```python
from build123d import *

# Parameters (mm, degrees)
BOSS_EXTRUDE2_DEPTH = 57.5
FILLET1_R           = 0.4
FILLET2_R           = 0.5
SKETCH5_R           = 4.25
CUT_EXTRUDE1_DEPTH  = 3
SKETCH6_R           = 3.25
CUT_EXTRUDE2_DEPTH  = 5.9
SKETCH7_R           = 4.25
CUT_EXTRUDE3_DEPTH  = 8
SKETCH8_R           = 3.25
CUT_EXTRUDE4_DEPTH  = 0.9
SKETCH9_W           = 30
SKETCH9_H           = 4.9
BOSS_EXTRUDE3_DEPTH = 2
CHAMFER1_SIZE       = 0.5


with BuildPart() as part:
    # Sketch4 → Boss-Extrude2 (new, symmetric)
    with BuildSketch(Plane(origin=(0, 0, 0), x_dir=(0, 0, -1), z_dir=(1, 0, 0))):
        Polygon((-15, 5), (15, 5), (15, 0.1), (5.883419246, 0.1), (8.770170592, -4.9), (-8.770170592, -4.9), (-5.883419246, 0.1), (-15, 0.1), align=None)
    extrude(amount=BOSS_EXTRUDE2_DEPTH, both=True)

    # Fillet1
    fillet1_edges = [part.edges().sort_by_distance(p)[0] for p in [
        (0, -4.9, -8.770170592),
        (0, -4.9, 8.770170592),
    ]]
    fillet(fillet1_edges, radius=FILLET1_R)

    # Fillet2
    fillet2_edges = [part.edges().sort_by_distance(p)[0] for p in [
        (0, 0.1, -5.883419246),
        (0, 0.1, 5.883419246),
    ]]
    fillet(fillet2_edges, radius=FILLET2_R)

    # Sketch5 → Cut-Extrude1 (cut)
    with BuildSketch(Plane.XZ.offset(4.9)):
        with Locations(Location((51.5, 0, 0), (0, 0, 270))):
            Circle(SKETCH5_R)
    extrude(amount=-CUT_EXTRUDE1_DEPTH, mode=Mode.SUBTRACT)

    # Sketch6 → Cut-Extrude2 (cut)
    with BuildSketch(Plane(origin=(0, 5, 0), x_dir=(1, 0, 0), z_dir=(0, 1, 0))):
        with Locations(Location((51.5, 0, 0), (0, 0, 270))):
            Circle(SKETCH6_R)
    extrude(amount=-CUT_EXTRUDE2_DEPTH, mode=Mode.SUBTRACT)

    # Sketch7 → Cut-Extrude3 (cut)
    with BuildSketch(Plane.XZ.offset(4.9)):
        with Locations(Location((-51.5, 0, 0), (0, 0, 270))):
            Circle(SKETCH7_R)
    extrude(amount=-CUT_EXTRUDE3_DEPTH, mode=Mode.SUBTRACT)

    # Sketch8 → Cut-Extrude4 (cut)
    with BuildSketch(Plane(origin=(0, 5, 0), x_dir=(1, 0, 0), z_dir=(0, 1, 0))):
        with Locations(Location((-51.5, 0, 0), (0, 0, 270))):
            Circle(SKETCH8_R)
    extrude(amount=-CUT_EXTRUDE4_DEPTH, mode=Mode.SUBTRACT)

    # Sketch9 → Boss-Extrude3 (add)
    with BuildSketch(Plane(origin=(57.5, 0, 0), x_dir=(0, 0, -1), z_dir=(1, 0, 0))):
        with Locations((0, 2.55)):
            Rectangle(SKETCH9_W, SKETCH9_H)
    extrude(amount=BOSS_EXTRUDE3_DEPTH)

    # Chamfer1
    chamfer1_edges = [part.edges().sort_by_distance(p)[0] for p in [
        (51.5, -4.9, 4.25),
        (-51.5, -4.9, 4.25),
    ]]
    chamfer(chamfer1_edges, length=CHAMFER1_SIZE)


solid = part.part
```
Could you check a few things on this model? Use its own coordinates, in mm. A direction names the side the tool comes from. Coordinates: 2 decimals unless noted, no trailing zeros. Write each loop counter-clockwise with the first axis right and the second up, starting at its lowest first coordinate (ties: lowest second). Pieces come first, ordered by that corner, then holes. Notation, with made-up numbers: (46.25, 7.5) - (82.25, 7.5) arc R21 ccw to (82.25, 31.5) - close; hole circle Ø11 at (5, 51). An arc over 180 degrees is marked (long way). Use a Markdown table: item, result.
Q1. Imagine slicing it at C-C (x = -51.5). List the corners of the cut face in (y, z) for me.
Geometry check:
| item | result |
|---|---|
| outline | (-4.9, -8.08) arc R0.4 ccw to (-4.3, -8.42) - (-0.65, -6.32) arc R0.5 cw to (0.1, -6.75) - (0.1, -15) - (5, -15) - (5, -3.25) - (4.1, -3.25) - (4.1, 3.25) - (5, 3.25) - (5, 15) - (0.1, 15) - (0.1, 6.75) arc R0.5 cw to (-0.65, 6.32) - (-4.3, 8.42) arc R0.4 ccw to (-4.9, 8.08) - (-4.9, 4.75) - (-4.4, 4.25) - (3.1, 4.25) - (3.1, -4.25) - (-4.4, -4.25) - (-4.9, -4.75) - close |
Q2. I'm going to push flat-ended pins straight in: pin 1 Ø7.5 at (x, z) = (-51.5, 0) entering from -Y; pin 2 Ø2 at (x, z) = (50, 1) entering from +Y; pin 3 Ø5.5 at (y, z) = (-3, -3.5) entering from +X. Where does each tip first touch, or does it pass through?
Geometry check:
| item | result |
|---|---|
| pin 1 | stops at y = 3.1 |
| pin 2 | stops at y = -0.9 |
| pin 3 | stops at x = 57.5 |
Q3. Imagine slicing it at B-B (x = 30). List the corners of the cut face in (y, z) for me.
Geometry check:
| item | result |
|---|---|
| outline | (-4.9, -8.08) arc R0.4 ccw to (-4.3, -8.42) - (-0.65, -6.32) arc R0.5 cw to (0.1, -6.75) - (0.1, -15) - (5, -15) - (5, 15) - (0.1, 15) - (0.1, 6.75) arc R0.5 cw to (-0.65, 6.32) - (-4.3, 8.42) arc R0.4 ccw to (-4.9, 8.08) - close |
Q4. Imagine slicing it at A-A (z = 0). List the corners of the cut face in (x, y) for me.
Geometry check:
| item | result |
|---|---|
| outline | (-57.5, -4.9) - (-56.25, -4.9) - (-55.75, -4.4) - (-55.75, 3.1) - (-47.25, 3.1) - (-47.25, -4.4) - (-46.75, -4.9) - (46.75, -4.9) - (47.25, -4.4) - (47.25, -1.9) - (55.75, -1.9) - (55.75, -4.4) - (56.25, -4.9) - (57.5, -4.9) - (57.5, 0.1) - (59.5, 0.1) - (59.5, 5) - (54.75, 5) - (54.75, -0.9) - (48.25, -0.9) - (48.25, 5) - (-48.25, 5) - (-48.25, 4.1) - (-54.75, 4.1) - (-54.75, 5) - (-57.5, 5) - close |
Q5. Please list where these lines run through material, in increasing order: L1, parallel to X at y = 0.9, z = 0; L2, parallel to X at y = -3.4, z = 0; L3, parallel to Y at x = 34, z = 12.25.
Geometry check:
| item | result |
|---|---|
| L1 | x = -57.5 to -55.75, -47.25 to 48.25, 54.75 to 59.5 |
| L2 | x = -57.5 to -55.75, -47.25 to 47.25, 55.75 to 57.5 |
| L3 | y = 0.1 to 5 |
Q6. Which directions (+Z, -Z, +X, -X, +Y, -Y) give clear straight access to the entire face, cutting with the end or side of a thin tool? Please do faces 1 (the flat face through (0.805, -2.449, -7.355)), 2 (the cylindrical face through (-54.673, 4.556, -0.705)), 3 (the cylindrical face through (-55.65, -0.7, 0.92)), 4 (the flat face through (57.5, -2, 0)).
Geometry check:
| item | result |
|---|---|
| face 1 | -Z, +X, -X |
| face 2 | +Y |
| face 3 | -Y |
| face 4 | +Z, -Z, +X, -Y |
Q7. Thinking about a two-plate mould opening in X: for faces 5 (the flat face through (52, -1.9, 0)), 6 (the flat face through (-51, 4.1, 0)), 7 (the flat face through (1, -4.9, 0)), 8 (the flat face through (59.5, 3, 0)), which applies, +X half, -X half, draft (parallel to the pull), parting line (faces both ways), or undercut?
Geometry check:
| item | result |
|---|---|
| face 5 | undercut |
| face 6 | undercut |
| face 7 | draft |
| face 8 | +X half |
Q8. Imagine slicing it at D-D (z = 10.5). List the corners of the cut face in (x, y) for me.
Geometry check:
| item | result |
|---|---|
| outline | (-57.5, 0.1) - (59.5, 0.1) - (59.5, 5) - (-57.5, 5) - close |
